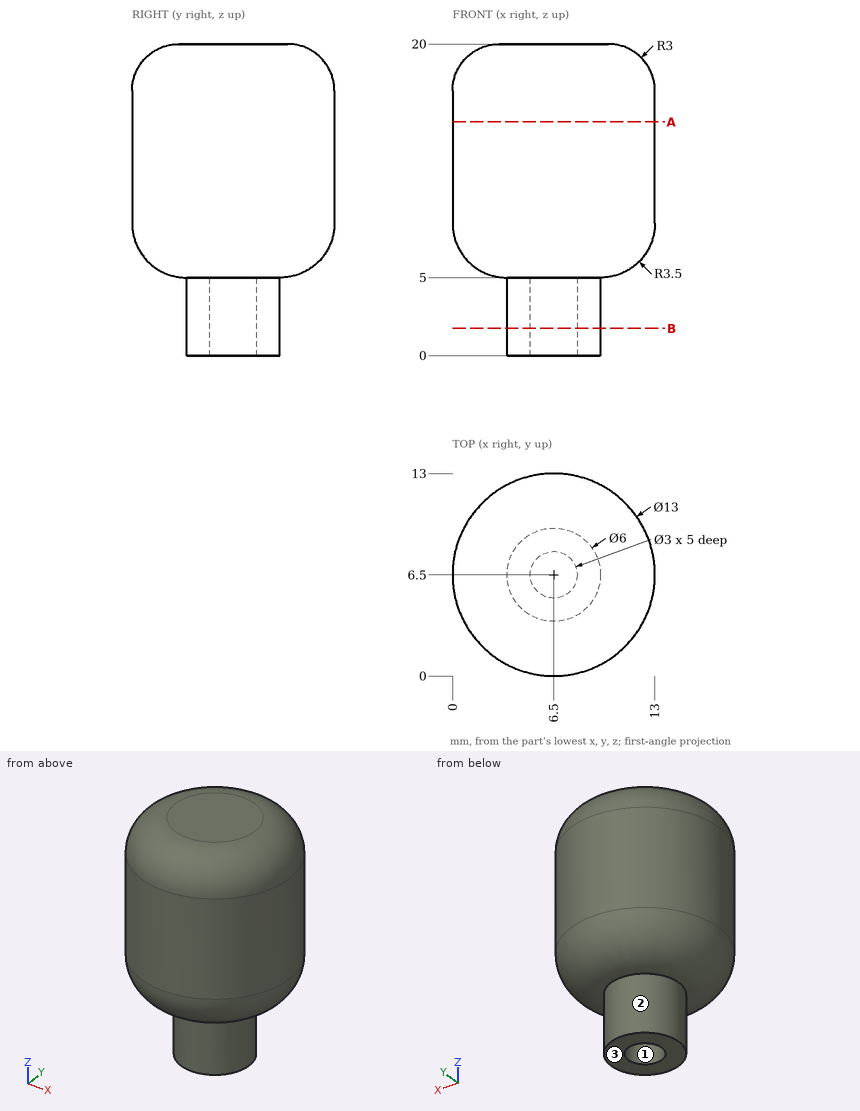
Could you check a few things on this drawing? It's one solid part, dimensions in mm from its lowest x, y, z. Round coordinates to 2 decimals unless told otherwise and drop trailing zeros. Write each loop counter-clockwise with the first axis right and the second up, starting at its lowest first coordinate (ties: lowest second). Pieces come first, ordered by that corner, then holes. Notation, with made-up numbers: (-11, 82.5) -> (18, 82.5) arc R17 ccw to (18, 91.5) -> close; hole circle Ø7 at (48, 32). An arc over 180 degrees is marked (long way). One line per question, with ' | ' between items. Start each with the question number.
1) I'm going to push flat-ended pins straight in: P1, Ø0.9, axis at x = 6, y = 6.5, coming from the -Z side; P2, Ø1.5, axis at x = 2, z = 16.5, coming from the +Y side; P3, Ø2, axis at x = 11.5, y = 10.5, coming from the -Z side. Where does each tip first touch, or does it pass through?
2) If we mould it in two halves opening along Y, with no side actions, what happens to the marked faces 1, 2 and 3? For each: released by +Y, released by -Y, zero draft, split by the parting line, or undercut.
3) Suppose I cut it at A-A on z = 15. Write out the boundary of the cut face in (x, y).
4) Suppose I cut it at B-B on z = 1.75. Write out the boundary of the cut face in (x, y), then the cut area to 3 significant figures.
5) I need wall thicknesses on line 1 (Y direction, x = 6.5, z = 3.85); line 2 (X direction, y = 5.25, z = 1.75). Which ranges of each line are inside material? Lowest first, please. Write a range as [from, to].
Return value:
1) P1: stops at z = 5 | P2: stops at y = 11.81 | P3: stops at z = 5.96
2) face 1: undercut | face 2: split by the parting line | face 3: zero draft
3) outline: circle Ø13 at (6.5, 6.5)
4) outline: circle Ø6 at (6.5, 6.5); hole circle Ø3 at (6.5, 6.5) | area: 21.2 mm2
5) line 1: y = [3.5, 5], [8, 9.5] | line 2: x = [3.77, 5.67], [7.33, 9.23]
